from build123d import *

# Parameters (mm, degrees)
EXTRUDE_1_DEPTH          = 51
SKETCH_2_R               = 1
CUT_EXTRUDE_1_DEPTH      = 51
SKETCH_3_R               = 1
CUT_EXTRUDE_2_DEPTH      = 51
MIRROR_3_COPY_1_SKETCH_R = 1
MIRROR_3_COPY_1_DEPTH    = 51
SKETCH_4_W               = 15
SKETCH_4_H               = 15
EXTRUDE_2_DEPTH          = 10


with BuildPart() as part:
    # 草图1 → 凸台-拉伸1 (new body)
    with BuildSketch(Plane(origin=(0, 0, 0), x_dir=(1, 0, 0), z_dir=(0, 1, 0))):
        Polygon((43.65, -94.842931951), (65.75, -9.25), (106.567585168, -9.25), (106.567585168, 9.25), (65.75, 9.25), (43.65, 94.842931951), (66.809562052, 122.798714511), (56.259562052, 131.538708791), (33.1, 103.58292623), (-33.1, 103.58292623), (-56.259562052, 131.538708791), (-66.809562052, 122.798714511), (-43.65, 94.842931951), (-65.75, 9.25), (-106.567585168, 9.25), (-106.567585168, -9.25), (-65.75, -9.25), (-43.65, -94.842931951), (-66.809562052, -122.798714511), (-56.259562052, -131.538708791), (-33.1, -103.58292623), (33.1, -103.58292623), (56.259562052, -131.538708791), (66.809562052, -122.798714511), align=None)
    extrude(amount=EXTRUDE_1_DEPTH)

    # 草图2 → 切除-拉伸1 (cut)
    with BuildSketch(Plane.XZ):
        with Locations((98.067585168, 0)):
            Circle(SKETCH_2_R)
    cut_extrude_1 = extrude(amount=-CUT_EXTRUDE_1_DEPTH, mode=Mode.SUBTRACT)

    # 镜向1: 切除-拉伸1 across plane
    add(cut_extrude_1.mirror(Plane(origin=(0, 0, 0), x_dir=(0, 0, 1), z_dir=(1, 0, 0))), mode=Mode.SUBTRACT)

    # 草图3 → 切除-拉伸2 (cut)
    with BuildSketch(Plane.XZ):
        with Locations((56.111937864, 120.623091213)):
            Circle(SKETCH_3_R)
    cut_extrude_2 = extrude(amount=-CUT_EXTRUDE_2_DEPTH, mode=Mode.SUBTRACT)

    # 镜向2: 切除-拉伸2 across plane
    add(cut_extrude_2.mirror(Plane(origin=(0, 0, 0), x_dir=(0, 0, 1), z_dir=(1, 0, 0))), mode=Mode.SUBTRACT)

    # 镜向3: 切除-拉伸2 across plane
    add(cut_extrude_2.mirror(Plane.XY), mode=Mode.SUBTRACT)

    # 镜向3 copy 1 sketch → 镜向3 copy 1 (cut)
    with BuildSketch(Plane(origin=(0, 0, 0), x_dir=(-1, 0, 0), z_dir=(0, -1, 0))):
        with Locations((56.111937864, 120.623091213)):
            Circle(MIRROR_3_COPY_1_SKETCH_R)
    extrude(amount=-MIRROR_3_COPY_1_DEPTH, mode=Mode.SUBTRACT)

    # 草图4 → 凸台-拉伸2 (add)
    with BuildSketch(Plane.XZ.offset(-51)):
        with Locations((0, 85.462689848)):
            Rectangle(SKETCH_4_W, SKETCH_4_H)
    extrude(amount=-EXTRUDE_2_DEPTH)


solid = part.part
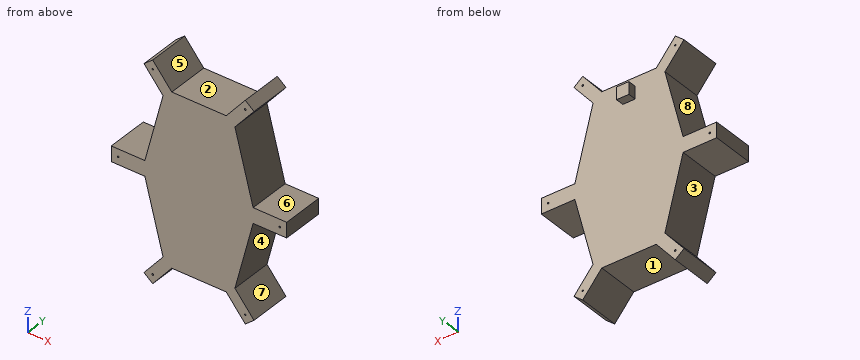
Can you work these out from the model? Positions are in its coordinate system, mm. Face numbers are marked on the shaded views. A direction names the side the tool comes from. Coordinates: 2 decimals unless noted, no trailing zeros. Write each loop counter-clockwise with the first axis right and the second up, starting at its lowest first coordinate (ties: lowest second). Pieces come first, ordered by that corner, then holes. Notation, with made-up numbers: (85, -34) -> (138, -34) arc R14 cw to (138, -20) -> close; hole circle Ø11 at (69, 68.25). An arc over 180 degrees is marked (long way). Write item = value, one per line.
(1) Imagine slicing it at C-C (z = -85). Please give me the cut outline in (x, y), and give its area (3 significant figures).
Verdict:
outline = (-46.19, 0) -> (46.19, 0) -> (46.19, 51) -> (-46.19, 51) -> close
area = 4,710 mm^2
(2) Thinking about a two-plate mould opening in X: for the marked faces 5, 6, 7 and 8, which applies, +X half, -X half, draft (parallel to the pull), parting line (faces both ways), or undercut?
Verdict:
face_5 = undercut
face_6 = draft
face_7 = +X half
face_8 = -X half
(3) Imagine slicing it at A-A (y = 17). State how many separate pieces and enclosed holes the cut face has, and give its area (3 significant figures).
Verdict:
separate_pieces = 1
enclosed_holes = 6
area = 26,000 mm^2
(4) On a 3-axis mill with a long thin cutter (end or side, diameter ignored), from which of +Z, -Z, +X, -X, +Y, -Y can I reach the whole of each face in a straight line? I mean the marked faces 1, 2, 3 and 4. Say none if no direction works.
Verdict:
face_1 = -Z, +Y, -Y
face_2 = +Z, +Y, -Y
face_3 = -X, +Y, -Y
face_4 = +X, +Y, -Y
(5) For pin 1 (10 mm diameter, centred on y = 45, z = 71, fed in from +X); pin 2 (1 mm diameter, centred on x = -6, z = -102.5, fed in from +Y); pin 3 (5 mm diameter, centred on y = 22, z = 62, fed in from +X); pin 4 (1.6 mm diameter, centred on x = 56.11, z = -120.62, fed in from -Y), each with a flat end and sliding along its axis, tell me the tip position at first contact or that it passes through.
Verdict:
pin_1 = 51.1
pin_2 = 51
pin_3 = 52.78
pin_4 = through
(6) Imagine slicing it at B-B (x = -1). Please give me the cut outline in (y, z).
Verdict:
outline = (0, -103.58) -> (51, -103.58) -> (51, 77.96) -> (61, 77.96) -> (61, 92.96) -> (51, 92.96) -> (51, 103.58) -> (0, 103.58) -> close
(7) Imagine slicing it at D-D (x = -86). Please give me the cut outline in (y, z), and give its area (4 significant figures).
Verdict:
outline = (0, -9.25) -> (51, -9.25) -> (51, 9.25) -> (0, 9.25) -> close
area = 943.5 mm^2
(8) If I drill on probe 1 along Y at (x, z) = (-23, 40); probe 2 along Z at (x, y) = (93, 50); probe 3 along Z at (x, y) = (8, 27.5), over which ranges is the centre line in solid material (lowest first)?
Verdict:
probe_1 = 0 to 51
probe_2 = -9.25 to 9.25
probe_3 = -103.58 to 103.58
